Verification items for this drawing (mm, ordinates from the low corner). Round coordinates to 2 decimals unless told otherwise and drop trailing zeros. Loops run counter-clockwise (first coordinate to the right, second up) from the corner with the lowest first, then second, coordinate; pieces in that order, holes last. Notation, with made-up numbers: M -6,-7.75 L 16,-7.75 A13 ccw 16,4.25 Z; hole C -7,-16 d1. An arc over 180 degrees is marked long. Use one line per item in the form item = value. Start each with the question number.
1. Cross-section at B-B (z = 9). Record the boundary of the cut face in (x, y), then the cut area to 3 significant figures.
2. Cross-section at C-C (z = 41). Record the boundary of the cut face in (x, y).
3. Cross-section at A-A (x = 7). Record the boundary of the cut face in (y, z), then the cut area to 3 significant figures.
4. Draft check along Z on the marked faces 1, 2, 3 and 4. Enter one of: pulls with the +Z half, pulls with the -Z half, needs draft (parallel to the pull), parting line crosses it, or undercut.
5. Go/stop test with flat-tipped pins: pin 1 (1.5 mm diameter, centred on x = 17.5, z = 42.5, fed in from +Y); pin 2 (3.5 mm diameter, centred on x = 7.5, z = 58, fed in from -Y); pin 3 (1.8 mm diameter, centred on x = 65, z = 9, fed in from -Y). Record where each tip stops, or that it passes through.
6. Material ranges on line 1 (Z direction, x = 71, y = 28.9); line 2 (Z direction, x = 65, y = 4.35); line 3 (Z direction, x = 31, y = 33.5), recorded low to high.
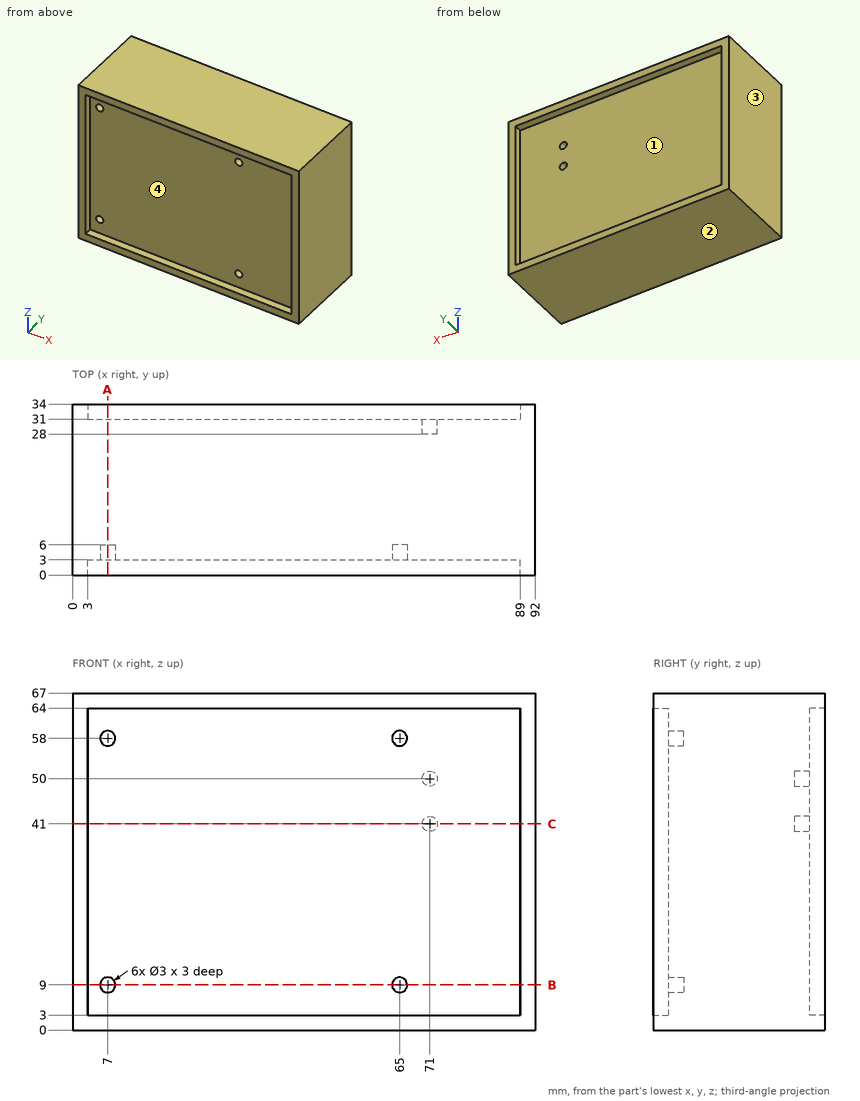
Reported:
q1.outline = M 0,0 L 3,0 L 3,3 L 5.5,3 L 5.5,6 L 8.5,6 L 8.5,3 L 63.5,3 L 63.5,6 L 66.5,6 L 66.5,3 L 89,3 L 89,0 L 92,0 L 92,34 L 89,34 L 89,31 L 3,31 L 3,34 L 0,34 Z
q1.area = 2,590 mm²
q2.outline = M 0,0 L 3,0 L 3,3 L 89,3 L 89,0 L 92,0 L 92,34 L 89,34 L 89,31 L 72.5,31 L 72.5,28 L 69.5,28 L 69.5,31 L 3,31 L 3,34 L 0,34 Z
q3.outline = M 0,0 L 34,0 L 34,3 L 31,3 L 31,64 L 34,64 L 34,67 L 0,67 L 0,64 L 3,64 L 3,59.5 L 6,59.5 L 6,56.5 L 3,56.5 L 3,10.5 L 6,10.5 L 6,7.5 L 3,7.5 L 3,3 L 0,3 Z
q3.area = 1,890 mm²
q4.face_1 = undercut
q4.face_2 = pulls with the -Z half
q4.face_3 = needs draft
q4.face_4 = undercut
q5.pin_1 = 31
q5.pin_2 = 3
q5.pin_3 = 6
q6.line_1 = 0 to 39.5, 42.5 to 48.5, 51.5 to 67
q6.line_2 = 0 to 7.5, 10.5 to 56.5, 59.5 to 67
q6.line_3 = 0 to 3, 64 to 67
